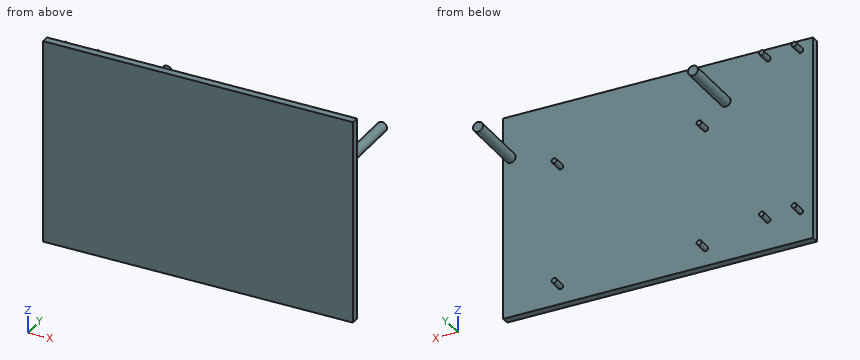
```python
from build123d import *

# Parameters (mm, degrees)
SKETCH7_W           = 124
SKETCH7_H           = 82
BOSS_EXTRUDE3_DEPTH = 3
SKETCH8_R           = 2
BOSS_EXTRUDE4_DEPTH = 25
SKETCH9_R           = 1
BOSS_EXTRUDE5_DEPTH = 5
SKETCH10_R          = 1
BOSS_EXTRUDE6_DEPTH = 5


with BuildPart() as part:
    # Sketch7 → Boss-Extrude3 (new body)
    with BuildSketch(Plane(origin=(0, 0, 0), x_dir=(1, 0, 0), z_dir=(0, 1, 0))):
        Rectangle(SKETCH7_W, SKETCH7_H)
    extrude(amount=BOSS_EXTRUDE3_DEPTH)

    # Sketch8 → Boss-Extrude4 (add)
    with BuildSketch(Plane(origin=(0, 3, 0), x_dir=(1, 0, 0), z_dir=(0, 1, 0))):
        with Locations(Location((59, -24, 0), (0, 0, 90))):
            Circle(SKETCH8_R)
        with Locations(Location((-27, -24, 0), (0, 0, 90))):
            Circle(SKETCH8_R)
    extrude(amount=BOSS_EXTRUDE4_DEPTH)

    # Sketch9 → Boss-Extrude5 (add)
    with BuildSketch(Plane(origin=(0, 3, 0), x_dir=(1, 0, 0), z_dir=(0, 1, 0))):
        with Locations(Location((39, 34, 0), (0, 0, 90))):
            Circle(SKETCH9_R)
        with Locations(Location((-19, 34, 0), (0, 0, 90))):
            Circle(SKETCH9_R)
        with Locations(Location((-19, -15, 0), (0, 0, 90))):
            Circle(SKETCH9_R)
        with Locations(Location((39, -15, 0), (0, 0, 90))):
            Circle(SKETCH9_R)
    extrude(amount=BOSS_EXTRUDE5_DEPTH)

    # Sketch10 → Boss-Extrude6 (add)
    with BuildSketch(Plane(origin=(0, 3, 0), x_dir=(1, 0, 0), z_dir=(0, 1, 0))):
        with Locations(Location((-57, -37, 0), (0, 0, 90))):
            Circle(SKETCH10_R)
        with Locations(Location((-44, -37, 0), (0, 0, 90))):
            Circle(SKETCH10_R)
        with Locations(Location((-44, 29, 0), (0, 0, 90))):
            Circle(SKETCH10_R)
        with Locations(Location((-57, 29, 0), (0, 0, 90))):
            Circle(SKETCH10_R)
    extrude(amount=BOSS_EXTRUDE6_DEPTH)


solid = part.part
```
Build history of the part. All positions in model axes, mm. Coordinates: 2 decimals unless noted, no trailing zeros. Order: outer loops, then holes, each group sorted by start corner. A loop starts at its lowest first (then second) coordinate and runs counter-clockwise, first axis right, second up. Notation, with made-up numbers: (85.25, 67.5) -> (118.25, 67.5) arc R15 cw to (118.25, 85.5) -> close; hole circle Ø4 at (88, 20). An arc over 180 degrees is marked (long way). Answer in a Markdown table with one row per item. Add a question column.
Q1. Drop flat-ended pins along their axis: pin 1 (12 mm diameter, centred on y = 11.5, z = 22, fed in from -X); pin 2 (2 mm diameter, centred on y = 11, z = 22, fed in from -X); pin 3 (1.6 mm diameter, centred on x = 39, z = -34, fed in from +Y). Give the stop position or say it passes through.
Q2. Band-saw the part on B-B, the plane z = 24. List the corners of the cut face in (x, y).
Q3. Band-saw the part on A-A, the plane y = 22. List the corners of the cut face in (x, z), then the cut area to 3 significant figures.
Q4. Wall check: line 1 along Y through (x, z) = (17.5, 25.5); line 2 along Z through (x, y) = (-28.5, 3.5). Give the ranges that are in metal, low to high. Write a range as [from, to].
Q5. Band-saw the part on D-D, the plane z = 33. List the corners of the cut face in (x, y), then the cut area to 3 significant figures.
Q6. Band-saw the part on C-C, the plane x = 19. List the corners of the cut face in (y, z).
Answers follow:
| question | item | result |
|---|---|---|
| 1 | pin 1 | x = -29 |
| 1 | pin 2 | x = -28.73 |
| 1 | pin 3 | y = 8 |
| 2 | outline | (-62, 0) -> (62, 0) -> (62, 3) -> (61, 3) -> (61, 28) -> (57, 28) -> (57, 3) -> (-25, 3) -> (-25, 28) -> (-29, 28) -> (-29, 3) -> (-62, 3) -> close |
| 3 | outline | circle Ø4 at (-27, 24); circle Ø4 at (59, 24) |
| 3 | area | 25.1 mm^2 |
| 4 | line 1 | [0, 3] |
| 4 | line 2 | [22.68, 25.32] |
| 5 | outline | (-62, 0) -> (62, 0) -> (62, 3) -> (-62, 3) -> close |
| 5 | area | 372 mm^2 |
| 6 | outline | (0, -41) -> (3, -41) -> (3, 41) -> (0, 41) -> close |
